CAD build for the part. Positions are in the model's coordinates, mm. Round coordinates to 2 decimals unless told otherwise and drop trailing zeros. Loops run counter-clockwise (first coordinate to the right, second up) from the corner with the lowest first, then second, coordinate; pieces in that order, holes last.
```python
from build123d import *

# Parameters (mm, degrees)
SKETCH1_W           = 75
SKETCH1_H           = 20
SKETCH1_R           = 4.9
BOSS_EXTRUDE1_DEPTH = 20
FILLET1_R           = 10


with BuildPart() as part:
    # Sketch1 → Boss-Extrude1 (new, symmetric)
    with BuildSketch(Plane(origin=(0, 0, 0), x_dir=(0, 0, -1), z_dir=(1, 0, 0))):
        Rectangle(SKETCH1_W, SKETCH1_H)
        with Locations((-25, 0)):
            Circle(SKETCH1_R, mode=Mode.SUBTRACT)
        with Locations((25, 0)):
            Circle(SKETCH1_R, mode=Mode.SUBTRACT)
    extrude(amount=BOSS_EXTRUDE1_DEPTH, both=True)

    # Fillet1
    fillet1_edges = [part.edges().sort_by_distance(p)[0] for p in [
        (0, 10, 37.5),
        (0, 10, -37.5),
    ]]
    fillet(fillet1_edges, radius=FILLET1_R)


solid = part.part
```
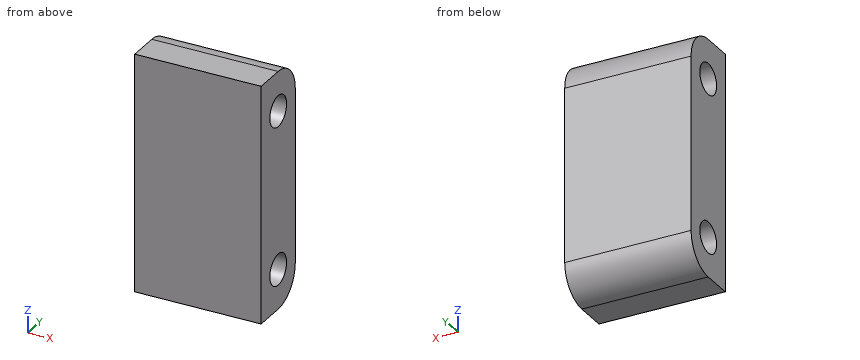
Item 1: Cut at C-C, the plane y = 6.75. Give the cut face in (x, z).
Answers follow:
outline: (-20, -34.88) - (20, -34.88) - (20, 34.88) - (-20, 34.88) - close
Item 2: Flat gauge pins, fed straight in: P1, Ø1, axis at x = 1.5, y = 7.5, coming from the +Z side; P2, Ø8, axis at x = 9, y = 6, coming from the +Z side. Where does each tip first touch, or does it go through?
Answers follow:
P1: stops at z = 34.64
P2: stops at z = 37.3
Item 3: Cut at B-B, the plane x = 5.5. Give the cut face in (y, z).
Answers follow:
outline: (-10, -37.5) - (0, -37.5) arc R10 ccw to (10, -27.5) - (10, 27.5) arc R10 ccw to (0, 37.5) - (-10, 37.5) - close; hole circle Ø9.8 at (0, -25); hole circle Ø9.8 at (0, 25)
Item 4: Probe line 1 (Y direction, x = 7, z = -25); line 2 (Z direction, x = -7.5, y = 3); line 3 (Z direction, x = 11, y = -0.75). List the from-to ranges inside material, lowest first.
Answers follow:
line 1: y = -10 to -4.9, 4.9 to 10
line 2: z = -37.04 to -28.87, -21.13 to 21.13, 28.87 to 37.04
line 3: z = -37.5 to -29.84, -20.16 to 20.16, 29.84 to 37.5
Item 5: Cut at A-A, the plane z = 25. Give the cut face in (x, y), plus the area to 3 significant figures.
Answers follow:
outline: (-20, -10) - (20, -10) - (20, -4.9) - (-20, -4.9) - close; (-20, 4.9) - (20, 4.9) - (20, 10) - (-20, 10) - close
area: 408 mm2
